Check sheet for the modelled part. Datum: model origin and axes. Units: mm. A direction names the side the tool comes from. Give positions to 0.01 mm unless a question says otherwise; leave off trailing zeros. Order: outer loops, then holes, each group sorted by start corner. A loop starts at its lowest first (then second) coordinate and runs counter-clockwise, first axis right, second up. Notation, with made-up numbers: M 8.5,71 L 48.5,71 A32 cw 48.5,100 Z; hole C 37,63.5 d2. An arc over 180 degrees is marked long. Return JSON: item names as keys, results as strings. Group by question number.
from build123d import *

# Parameters (mm, degrees)
ESBO_O1_W                = 184
ESBO_O1_H                = 136
RESSALTO_EXTRUS_O1_DEPTH = 2
ESBO_O2_W                = 184
ESBO_O2_H                = 136
ESBO_O2_W_2              = 180
ESBO_O2_H_2              = 132
EXTRUS_O_FINA1_DEPTH     = 65
CORTE_EXTRUS_O1_DEPTH    = 178.338659068


with BuildPart() as part:
    # Esboço1 → Ressalto-extrusão1 (new body)
    with BuildSketch(Plane(origin=(0, 0, 0), x_dir=(1, 0, 0), z_dir=(0, 1, 0))):
        Rectangle(ESBO_O1_W, ESBO_O1_H)
    extrude(amount=RESSALTO_EXTRUS_O1_DEPTH)

    # Esboço2 → Extrusão-Fina1 (add)
    with BuildSketch(Plane(origin=(0, 2, 0), x_dir=(1, 0, 0), z_dir=(0, 1, 0))):
        Rectangle(ESBO_O2_W, ESBO_O2_H)
        Rectangle(ESBO_O2_W_2, ESBO_O2_H_2, mode=Mode.SUBTRACT)
    extrude(amount=EXTRUS_O_FINA1_DEPTH)

    # Esboço3 → Corte-extrusão1 (cut, through all)
    with BuildSketch(Plane.XY.offset(68)):
        with BuildLine():
            Line((-25, 38.5), (25, 38.5))
            ThreePointArc((25, 38.5), (30, 33.5), (25, 28.5))
            Line((25, 28.5), (-25, 28.5))
            ThreePointArc((-25, 28.5), (-30, 33.5), (-25, 38.5))
        make_face()
    extrude(amount=-CORTE_EXTRUS_O1_DEPTH, mode=Mode.SUBTRACT)


solid = part.part
1) Sectioned sample at B-B on x = -43. Record the boundary of the cut face in (y, z).
2) Sectioned sample at C-C on z = 23. Record the boundary of the cut face in (x, y), then the cut area to 3 significant figures.
3) Tool access check on faces 4 (the face through (-30, 33.4, -67)), 5 (the face through (90, 34, 1)), 6 (the face through (-1, 0, -1)). Record the directions out of +Z, -Z, +X, -X, +Y, -Y that give a thin tool (end or side, any length) a straight path to the whole face; none if there is none.
4) Release check for a two-part mould opening along Y. For faces 1 (the face through (-1, 2, -1)), 2 (the face through (-30, 33.4, 67)), 3 (the face through (-1, 27, 66)) record: released by +Y, released by -Y, zero draft, split by the parting line, or undercut.
5) Sectioned sample at A-A on y = 21. Record the boundary of the cut face in (x, z).
6) Material ranges on line 1 along Z through (x, y) = (42, 17); line 2 along X through (y, z) = (54, -1); line 3 along Y through (x, z) = (6, -22.5), recorded low to high.
Reply:
{
 "1": {"outline": "M 0,-68 L 67,-68 L 67,-66 L 2,-66 L 2,66 L 67,66 L 67,68 L 0,68 Z"},
 "2": {"outline": "M -92,0 L 92,0 L 92,67 L 90,67 L 90,2 L -90,2 L -90,67 L -92,67 Z", "area": "628 mm^2"},
 "3": {"face 4": "+Z, -Z", "face 5": "+Y", "face 6": "+Z, -Z, +X, -X, -Y"},
 "4": {"face 1": "released by +Y", "face 2": "undercut", "face 3": "zero draft"},
 "5": {"outline": "M -92,-68 L 92,-68 L 92,68 L -92,68 Z; hole M -90,-66 L 90,-66 L 90,66 L -90,66 Z"},
 "6": {"line 1": "-68 to -66, 66 to 68", "line 2": "-92 to -90, 90 to 92", "line 3": "0 to 2"}
}
